Design review of the part built by this model. Coordinates are the model's own, in mm. Coordinates: 2 decimals unless noted, no trailing zeros. Write each loop counter-clockwise with the first axis right and the second up, starting at its lowest first coordinate (ties: lowest second). Pieces come first, ordered by that corner, then holes.
Q1. Take a section at C-C, the plane z = -22. Write out the cut boundary in (x, y), plus the area to 3 significant figures.
Q2. Take a section at A-A, the plane z = 0. Write out the cut boundary in (x, y).
Q3. Take a section at D-D, the plane z = -30. Write out the cut boundary in (x, y).
Q4. For L1, parallel to X at y = 3.8, z = 0; L2, parallel to X at y = 0.3, z = -3; L3, parallel to Z at x = -17, y = 3.8, list the stretches that pass through material, from the lowest coordinate up.
Q5. For pin 1 Ø2.5 at (x, z) = (4.24, 4.24) entering from -Y; pin 2 Ø5.5 at (x, z) = (0, 0) entering from +Y; pin 3 Ø1 at (y, z) = (3.5, 9.5) entering from +X; pin 4 Ø2 at (x, y) = (11, 2) entering from -Z, all flat-tipped, find the tip position at first contact; note any pin that passes through.
Q6. Take a section at B-B, the plane x = 0. Write out the cut boundary in (y, z).
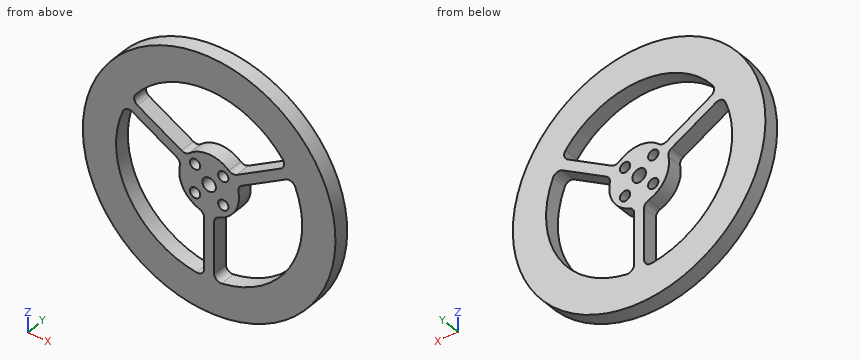
from build123d import *

# Parameters (mm, degrees)
SKETCH1_R           = 38
SKETCH1_R_2         = 28
BOSS_EXTRUDE1_DEPTH = 4.7
SKETCH2_R           = 9
SKETCH2_R_2         = 2.05
SKETCH2_R_3         = 1.55
BOSS_EXTRUDE2_DEPTH = 4.7
SKETCH3_W           = 3
SKETCH3_H           = 20.125880325
BOSS_EXTRUDE3_DEPTH = 4.7
FILLET1_R           = 2
FILLET2_R           = 2


with BuildPart() as part:
    # Sketch1 → Boss-Extrude1 (new body)
    with BuildSketch(Plane(origin=(0, 0, 0), x_dir=(1, 0, 0), z_dir=(0, 1, 0))):
        with Locations(Location((0, 0, 0), (0, 0, 270))):
            Circle(SKETCH1_R)
        with Locations(Location((0, 0, 0), (0, 0, 270))):
            Circle(SKETCH1_R_2, mode=Mode.SUBTRACT)
    extrude(amount=BOSS_EXTRUDE1_DEPTH)



with BuildPart() as body_2:
    # Sketch2 → Boss-Extrude2 (new body)
    with BuildSketch(Plane(origin=(0, 0, 0), x_dir=(1, 0, 0), z_dir=(0, 1, 0))):
        with Locations(Location((0, 0, 0), (0, 0, 270))):
            Circle(SKETCH2_R)
        with Locations(Location((0, 0, 0), (0, 0, 270))):
            Circle(SKETCH2_R_2, mode=Mode.SUBTRACT)
        with Locations(Location((-4.242640687, 4.242640687, 0), (0, 0, 270))):
            Circle(SKETCH2_R_3, mode=Mode.SUBTRACT)
        with Locations(Location((-4.242640687, -4.242640687, 0), (0, 0, 270))):
            Circle(SKETCH2_R_3, mode=Mode.SUBTRACT)
        with Locations(Location((4.242640687, -4.242640687, 0), (0, 0, 270))):
            Circle(SKETCH2_R_3, mode=Mode.SUBTRACT)
        with Locations(Location((4.242640687, 4.242640687, 0), (0, 0, 270))):
            Circle(SKETCH2_R_3, mode=Mode.SUBTRACT)
    extrude(amount=BOSS_EXTRUDE2_DEPTH)


with BuildPart() as part_1:
    add(part.part)

    add(body_2.part)  # Boss-Extrude3 merges body 2
    # Sketch3 → Boss-Extrude3 (add)
    with BuildSketch(Plane(origin=(0, 0, 0), x_dir=(1, 0, 0), z_dir=(0, 1, 0))):
        with Locations((0, 18.937059838)):
            Rectangle(SKETCH3_W, SKETCH3_H)
        Polygon((25.86473671, -13.200961894), (24.36473671, -15.799038106), (6.935213074, -5.736097943), (8.435213074, -3.138021732), align=None)
        Polygon((-24.36473671, -15.799038106), (-25.86473671, -13.200961894), (-8.435213074, -3.138021732), (-6.935213074, -5.736097943), align=None)
    extrude(amount=BOSS_EXTRUDE3_DEPTH)

    # Fillet1
    fillet1_edges = [part_1.edges().sort_by_distance(p)[0] for p in [
        (1.5, 2.35, -27.95979256),
        (-1.5, 2.35, -27.95979256),
        (24.963890642, 2.35, 12.680858174),
        (23.463890642, 2.35, 15.278934386),
        (-23.463890642, 2.35, 15.278934386),
        (-24.963890642, 2.35, 12.680858174),
    ]]
    fillet(fillet1_edges, radius=FILLET1_R)

    # Fillet2
    fillet2_edges = [part_1.edges().sort_by_distance(p)[0] for p in [
        (-1.5, 2.35, -8.874119675),
        (1.5, 2.35, -8.874119675),
        (8.435213074, 2.35, 3.138021732),
        (6.935213074, 2.35, 5.736097943),
        (-6.935213074, 2.35, 5.736097943),
        (-8.435213074, 2.35, 3.138021732),
    ]]
    fillet(fillet2_edges, radius=FILLET2_R)


solid = part_1.part
Responses:
1. outline: (-30.98, 0) - (-17.32, 0) - (-17.32, 4.7) - (-30.98, 4.7) - close; (-1.5, 0) - (1.5, 0) - (1.5, 4.7) - (-1.5, 4.7) - close; (17.32, 0) - (30.98, 0) - (30.98, 4.7) - (17.32, 4.7) - close
1. area: 143 mm2
2. outline: (-38, 0) - (-28, 0) - (-28, 4.7) - (-38, 4.7) - close; (-9, 0) - (-2.05, 0) - (-2.05, 4.7) - (-9, 4.7) - close; (2.05, 0) - (9, 0) - (9, 4.7) - (2.05, 4.7) - close; (28, 0) - (38, 0) - (38, 4.7) - (28, 4.7) - close
3. outline: (-23.32, 0) - (23.32, 0) - (23.32, 4.7) - (-23.32, 4.7) - close
4. L1: x = -38 to -28, -9 to -2.05, 2.05 to 9, 28 to 38
4. L2: x = -37.88 to -27.84, -8.49 to -5.17, -3.32 to 3.32, 5.17 to 8.49, 27.84 to 37.88
4. L3: z = -33.99 to -22.25, 8.08 to 11.55, 22.25 to 33.99
5. pin 1: passes through
5. pin 2: stops at y = 4.7
5. pin 3: stops at x = 36.92
5. pin 4: stops at z = -36.66
6. outline: (0, -38) - (4.7, -38) - (4.7, -2.05) - (0, -2.05) - close; (0, 2.05) - (4.7, 2.05) - (4.7, 9) - (0, 9) - close; (0, 28) - (4.7, 28) - (4.7, 38) - (0, 38) - close
